Study the drawing (mm; zero at the part's minimum x, y, z) and answer. A direction names the side the tool comes from. Round coordinates to 2 decimals unless told otherwise and drop trailing zeros. Write each loop counter-clockwise with the first axis right and the second up, starting at its lowest first coordinate (ties: lowest second). Pieces come first, ordered by that corner, then holes. Notation, with made-up numbers: M 37.5,15 L 73.5,15 A12 ccw 73.5,22 Z; hole C 33.25,-31.75 d1. An arc over 180 degrees is marked long. Put each result on its own line as item: value. Start each with the question number.
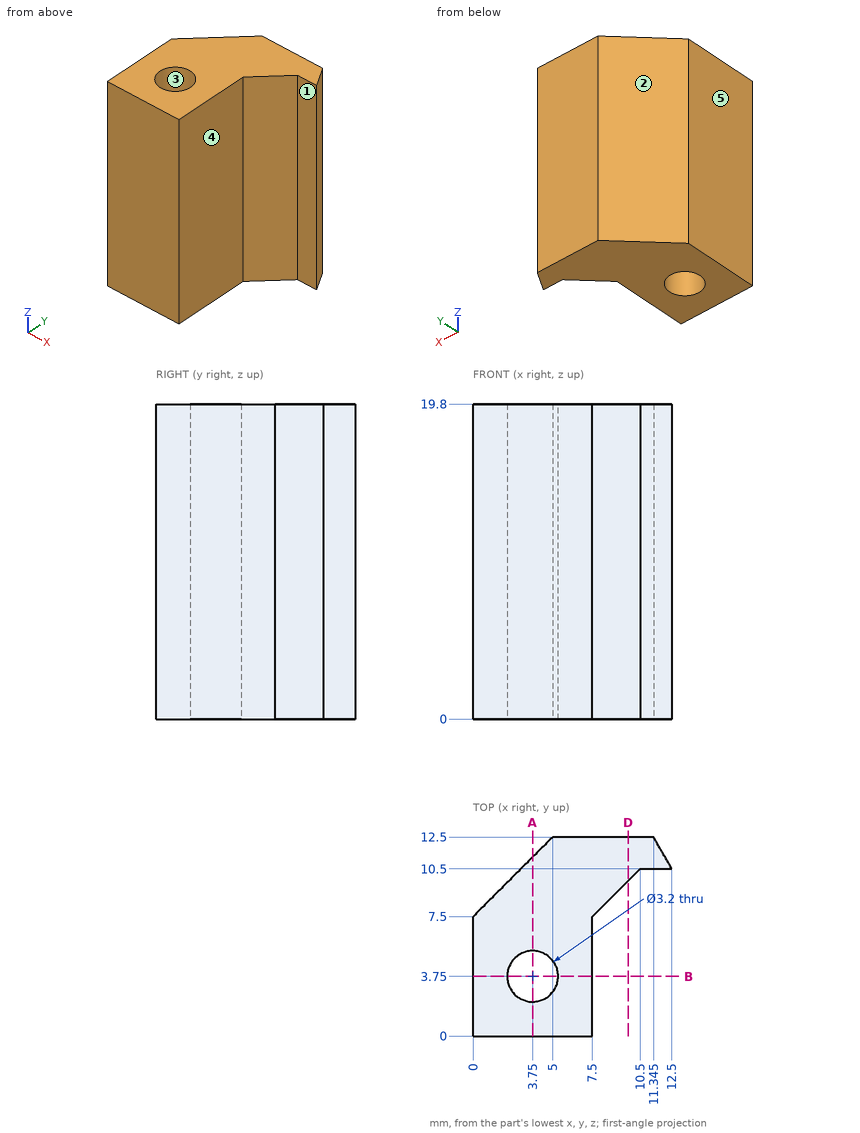
Item 1: Section A-A (x = 3.75) is taken. Give the vertices of the cut face in (y, z), and give its area (3 significant figures).
Item 2: Determine the mould class of the marked faces 1, 2 and 3 for opening direction X: released by +X, released by -X, zero draft, split by the parting line, or undercut.
Item 3: Section B-B (y = 3.75) is taken. Give the vertices of the cut face in (x, z).
Item 4: Consider line 1 along X through (y, z) = (6.5, 7.75); line 2 along X through (y, z) = (5, 6.25); line 3 along Y through (x, z) = (3.75, 15.75). Determine where each line is inside the solid, lowest interval first. Write a range as [from, to].
Item 5: Section D-D (x = 9.75) is taken. Give the vertices of the cut face in (y, z).
Item 6: Which of the six approach directions +Z, -Z, +X, -X, +Y, -Y give full straight-line access (tool end or side, diameter ignored) to the marked faces 4 and 5?
Output values:
1. outline: M 0,0 L 2.15,0 L 2.15,19.8 L 0,19.8 Z; M 5.35,0 L 11.25,0 L 11.25,19.8 L 5.35,19.8 Z
1. area: 159 mm^2
2. face 1: zero draft
2. face 2: released by -X
2. face 3: undercut
3. outline: M 0,0 L 2.15,0 L 2.15,19.8 L 0,19.8 Z; M 5.35,0 L 7.5,0 L 7.5,19.8 L 5.35,19.8 Z
4. line 1: x = [0, 7.5]
4. line 2: x = [0, 2.75], [4.75, 7.5]
4. line 3: y = [0, 2.15], [5.35, 11.25]
5. outline: M 9.75,0 L 12.5,0 L 12.5,19.8 L 9.75,19.8 Z
6. face 4: +Z, -Z, +X, -Y
6. face 5: +Z, -Z, -X, +Y, -Y
